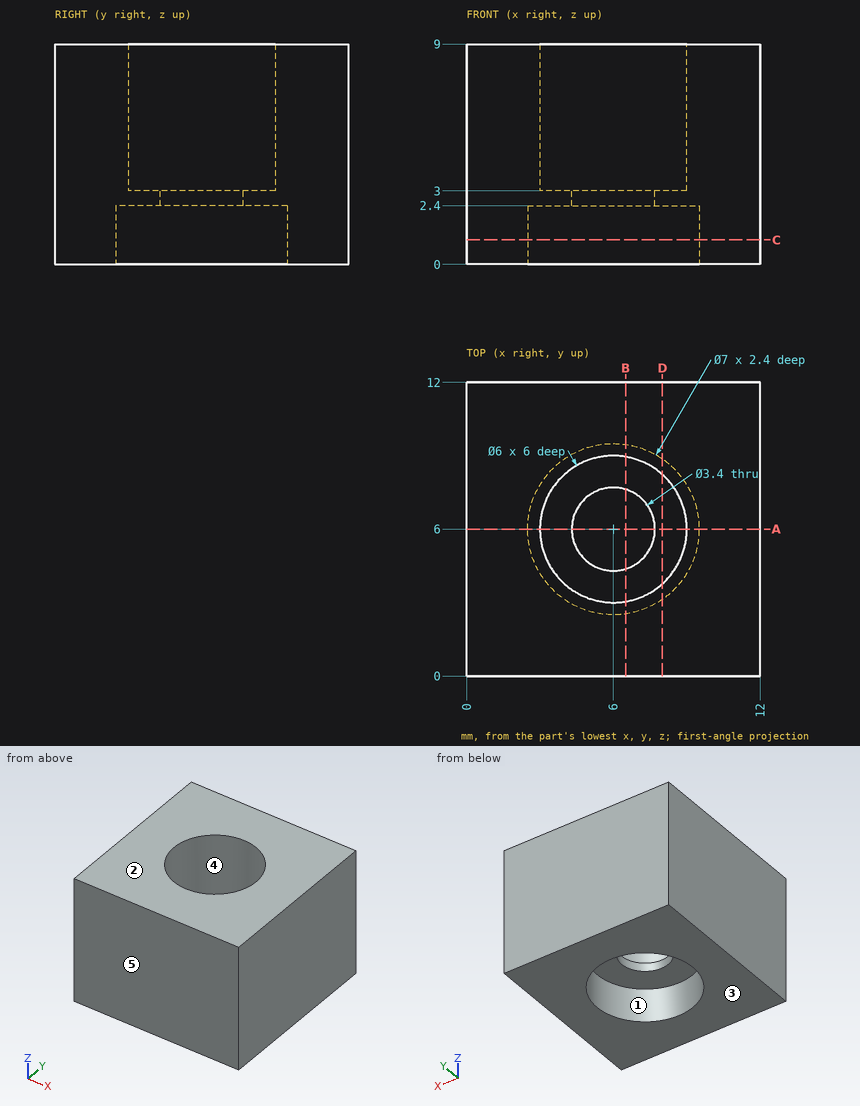
Geometry: see drawing. Coordinates: mm, zero at the bounding-box minimum. A direction names the side the tool comes from. Round coordinates to 2 decimals unless told otherwise and drop trailing zeros. Write each loop counter-clockwise with the first axis right and the second up, starting at its lowest first coordinate (ties: lowest second). Pieces come first, ordered by that corner, then holes.
1) Cut plane D-D (x = 8). Return the cut outline in (y, z).
2) Cut plane B-B (x = 6.5). Return the cut outline in (y, z).
3) Draft query along Y for the marked faces 3, 4 and 5. Return one class per face: pulls with the +Y half, pulls with the -Y half, needs draft (parallel to the pull), parting line crosses it, or undercut.
4) Cut plane A-A (y = 6). Return the cut outline in (x, z).
5) Ray query, L1, parallel to Y at x = 6, z = 2.75; L2, parallel to Y at x = 6, z = 5.3; L3, parallel to X at y = 3.25, z = 3.75. Return the intervals inside material, ascending.
6) Contact query for flat-ended pins moving along their axis: P1, Ø3, axis at x = 6, y = 6, coming from the -Z side; P2, Ø1, axis at x = 7, y = 7.5, coming from the +Z side. Output: stop coordinate, or through.
7) Reachability of the marked faces 1 and 2 from +Z, -Z, +X, -X, +Y, -Y: full face, straight path, thin tool, end or side. Return the list, or none.
8) Cut plane C-C (z = 1). Return the cut outline in (x, y), then the cut area to 3 significant figures.
Geometry says:
1. outline: (0, 0) - (3.13, 0) - (3.13, 2.4) - (8.87, 2.4) - (8.87, 0) - (12, 0) - (12, 9) - (8.24, 9) - (8.24, 3) - (3.76, 3) - (3.76, 9) - (0, 9) - close
2. outline: (0, 0) - (2.54, 0) - (2.54, 2.4) - (4.38, 2.4) - (4.38, 3) - (3.04, 3) - (3.04, 9) - (0, 9) - close; (7.62, 2.4) - (9.46, 2.4) - (9.46, 0) - (12, 0) - (12, 9) - (8.96, 9) - (8.96, 3) - (7.62, 3) - close
3. face 3: needs draft
3. face 4: undercut
3. face 5: pulls with the -Y half
4. outline: (0, 0) - (2.5, 0) - (2.5, 2.4) - (4.3, 2.4) - (4.3, 3) - (3, 3) - (3, 9) - (0, 9) - close; (7.7, 2.4) - (9.5, 2.4) - (9.5, 0) - (12, 0) - (12, 9) - (9, 9) - (9, 3) - (7.7, 3) - close
5. L1: y = 0 to 4.3, 7.7 to 12
5. L2: y = 0 to 3, 9 to 12
5. L3: x = 0 to 4.8, 7.2 to 12
6. P1: passes through
6. P2: stops at z = 3
7. face 1: -Z
7. face 2: +Z, +X, -X, +Y, -Y
8. outline: (0, 0) - (12, 0) - (12, 12) - (0, 12) - close; hole circle Ø7 at (6, 6)
8. area: 106 mm2
